Source: CAD feature listing. Evaluate the final solid. Frame: model axes, mm. Face numbers are marked on the shaded views. Give positions to 0.01 mm unless a question says otherwise; leave off trailing zeros. Order: outer loops, then holes, each group sorted by start corner. A loop starts at its lowest first (then second) coordinate and runs counter-clockwise, first axis right, second up. Notation, with made-up numbers: M 3,27.5 L 37,27.5 A29 ccw 37,58.5 Z; hole C 24,-9.75 d10. An arc over 180 degrees is marked long. Return JSON: item names as keys, results as strings.
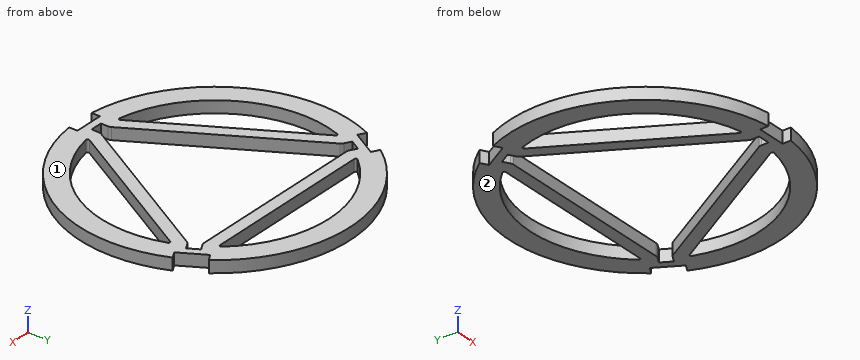
from build123d import *

# Parameters (mm, degrees)
BOSS_EXTRUDE1_DEPTH = 1.984375
FILLET1_R           = 0.25
FILLET2_R           = 1


with BuildPart() as part:
    # Sketch1 → Boss-Extrude1 (new body)
    with BuildSketch(Plane.XY):
        with BuildLine():
            Line((19.377158479, 8.437777007), (20.566763323, 9.124595684))
            ThreePointArc((20.566763323, 9.124595684), (19.485571585, -11.25), (2.38125, -22.373637354))
            Line((2.38125, -22.373637354), (2.38125, -21))
            Line((2.38125, -21), (-2.38125, -21))
            Line((-2.38125, -21), (-2.38125, -22.373637354))
            ThreePointArc((-2.38125, -22.373637354), (-19.485571585, -11.25), (-20.566763323, 9.124595684))
            Line((-20.566763323, 9.124595684), (-19.377158479, 8.437777007))
            Line((-19.377158479, 8.437777007), (-16.995908479, 12.562222993))
            Line((-16.995908479, 12.562222993), (-18.185513323, 13.24904167))
            ThreePointArc((-18.185513323, 13.24904167), (0, 22.5), (18.185513323, 13.24904167))
            Line((18.185513323, 13.24904167), (16.995908479, 12.562222993))
            Line((16.995908479, 12.562222993), (19.377158479, 8.437777007))
        make_face()
        with BuildLine():
            Line((-14.730919863, 12), (14.730919863, 12))
            ThreePointArc((14.730919863, 12), (0, 19), (-14.730919863, 12))
        make_face(mode=Mode.SUBTRACT)
        Polygon((-15.336133076, 10), (15.336133076, 10), (16.607907975, 10.73425958), (17.600095475, 9.01574042), (16.328320576, 8.281480839), (0.9921875, -18.281480839), (0.9921875, -19.75), (-0.9921875, -19.75), (-0.9921875, -18.281480839), (-16.328320576, 8.281480839), (-17.600095475, 9.01574042), (-16.607907975, 10.73425958), align=None, mode=Mode.SUBTRACT)
        with BuildLine():
            Line((-3.026844914, -18.757350822), (-17.757764777, 6.757350822))
            ThreePointArc((-17.757764777, 6.757350822), (-16.454482672, -9.5), (-3.026844914, -18.757350822))
        make_face(mode=Mode.SUBTRACT)
        with BuildLine():
            Line((17.757764777, 6.757350822), (3.026844914, -18.757350822))
            ThreePointArc((3.026844914, -18.757350822), (16.454482672, -9.5), (17.757764777, 6.757350822))
        make_face(mode=Mode.SUBTRACT)
    extrude(amount=BOSS_EXTRUDE1_DEPTH)

    # Fillet1
    fillet1_edges = [part.edges().sort_by_distance(p)[0] for p in [
        (14.730919863, 12, 0.9921875),
        (-14.730919863, 12, 0.9921875),
        (-17.757764777, 6.757350822, 0.9921875),
        (-3.026844914, -18.757350822, 0.9921875),
        (3.026844914, -18.757350822, 0.9921875),
        (17.757764777, 6.757350822, 0.9921875),
    ]]
    fillet(fillet1_edges, radius=FILLET1_R)

    # Fillet2
    fillet2_edges = [part.edges().sort_by_distance(p)[0] for p in [
        (15.336133076, 10, 0.9921875),
        (-15.336133076, 10, 0.9921875),
        (-16.328320576, 8.281480839, 0.9921875),
        (-0.9921875, -18.281480839, 0.9921875),
        (0.9921875, -18.281480839, 0.9921875),
        (16.328320576, 8.281480839, 0.9921875),
    ]]
    fillet(fillet2_edges, radius=FILLET2_R)


solid = part.part
1. Section query C-C (z = 0.9). State how many separate pieces and enclosed holes the cut face has, then the cut area to 3 significant figures.
Evaluation:
{"separate pieces": "1", "enclosed holes": "4", "area": "616 mm^2"}
2. First-contact query: pin 1 (2 mm diameter, centred on x = -3.5, y = 8.5, fed in from -Z); pin 2 (0.6 mm diameter, centred on y = -19, z = 1, fed in from -X); pin 3 (12 mm diameter, centred on x = 4.5, y = -17.5, fed in from -Z); pin 4 (0.6 mm diameter, centred on x = -0.5, z = 1.5, fed in from -Y). Flat tips, straight axial feed; report the tip coordinate or a pass-through.
Evaluation:
{"pin 1": "passes through", "pin 2": "stops at x = -12.51", "pin 3": "stops at z = 0", "pin 4": "stops at y = -21"}
3. Section query A-A (y = -8.5). Return loops of the section in (x, z).
Evaluation:
{"outline": "M -20.83,0 L -16.99,0 L -16.99,1.98 L -20.83,1.98 Z; M -8.95,0 L -6.64,0 L -6.64,1.98 L -8.95,1.98 Z; M 6.64,0 L 8.95,0 L 8.95,1.98 L 6.64,1.98 Z; M 16.99,0 L 20.83,0 L 20.83,1.98 L 16.99,1.98 Z"}
4. Section query B-B (x = -9.5). Return loops of the section in (y, z).
Evaluation:
{"outline": "M -20.4,0 L -16.45,0 L -16.45,1.98 L -20.4,1.98 Z; M -7.55,0 L -3.55,0 L -3.55,1.98 L -7.55,1.98 Z; M 10,0 L 12,0 L 12,1.98 L 10,1.98 Z; M 16.45,0 L 20.4,0 L 20.4,1.98 L 16.45,1.98 Z"}
5. Draft query along Z for the marked faces 1 and 2. Return one class per face: pulls with the +Z half, pulls with the -Z half, needs draft (parallel to the pull), parting line crosses it, or undercut.
Evaluation:
{"face 1": "pulls with the +Z half", "face 2": "pulls with the -Z half"}
6. Ray query, probe 1 along X at (y, z) = (-10.5, 1.6); probe 2 along Y at (x, z) = (-17.5, 1.7); probe 3 along X at (y, z) = (-7.5, 0.9). Return the intervals inside material, ascending.
Evaluation:
{"probe 1": "x = -19.9 to -15.84, -7.79 to -5.48, 5.48 to 7.79, 15.84 to 19.9", "probe 2": "y = -14.14 to -7.4, 6.31 to 8.96, 9.19 to 11.69, 12.85 to 14.14", "probe 3": "x = -21.21 to -17.46, -9.53 to -7.22, 7.22 to 9.53, 17.46 to 21.21"}
